Source: CAD feature listing. Evaluate the final solid. Frame: model axes, mm. A direction names the side the tool comes from. Round coordinates to 2 decimals unless told otherwise and drop trailing zeros. Order: outer loops, then holes, each group sorted by start corner. A loop starts at its lowest first (then second) coordinate and runs counter-clockwise, first axis right, second up. Notation, with made-up numbers: M 88,22.25 L 93,22.25 A7 cw 93,32.25 Z; hole C 25,62.5 d1. An arc over 180 degrees is marked long. Answer as CSV lines item,"result". Start each with the question number.
Item 1: Set-up query: faces 4 (the face through (-30, 17.25, -30)), 5 (the face through (22.03, 68.58, 14.04)), 6 (the face through (-16.856, 53.615, 8.767)). Return all of +Z, -Z, +X, -X, +Y, -Y with unobstructed straight access to the full face (end or side cutting, diameter ignored); none if empty.
Item 2: First-contact query: P1, Ø12, axis at x = 35.5, z = 49, coming from the -Y side; P2, Ø4, axis at y = 88.5, z = 22, coming from the -X side; P3, Ø5, axis at x = -16.5, z = 49, coming from the +Y side; P4, Ø3, axis at x = -8.5, y = 46, coming from the +Z side. Flat tips, straight axial feed; report the tip coordinate or a pass-through.
Item 3: Pull-direction query (X, two-part tool) for faces 1 (the face through (8, 128.25, 23)), 2 (the face through (7.1, 119.7, 22.4)), 3 (the face through (35.694, 36.026, -4.686)); classes: +X half, -X half, draft (parallel to the pull), parting line (faces both ways), or undercut.
Item 4: Line query: line 1 (Z direction, x = 0, y = 124) (3 decimals); line 2 (X direction, y = 50, z = 0). Output: solid intervals per line, ascending. Write a range as [from, to].
Item 5: Section query A-A on y = 45. Return the cut outline in (x, z).
from build123d import *

# Parameters (mm, degrees)
F2_R    = 3
F3_R    = 3
F4_SIZE = 1
F5_SIZE = 0.5


with BuildPart() as f1:
    # F0 (on Right) → F1 (revolve)
    with BuildSketch(Plane.YZ):
        Polygon((0, 70), (0, 19), (105.75, 19), (110.25, 23.5), (128.25, 23.5), (128.25, 26.125), (112.25, 26.125), (109.8, 28.575), (73.7, 28.575), (71.25, 26.125), (66.25, 26.125), (52.25, 36), (17.25, 36), (17.25, 70), align=None)
    revolve(axis=Axis((0, 37.063913, 0), (0, 1, 0)))

    # F2
    f2_edges = [f1.edges().sort_by_distance(p)[0] for p in [
        (0, 17.25, -36),
        (0, 66.25, -26.125),
        (0, 71.25, -26.125),
        (0, 112.25, -26.125),
    ]]
    fillet(f2_edges, radius=F2_R)

    # F3
    f3_edges = [f1.edges().sort_by_distance(p)[0] for p in [
        (0, 110.25, -23.5),
    ]]
    fillet(f3_edges, radius=F3_R)

    # F4
    f4_edges = [f1.edges().sort_by_distance(p)[0] for p in [
        (0, 17.25, -70),
    ]]
    chamfer(f4_edges, length=F4_SIZE)

    # F5
    f5_edges = [f1.edges().sort_by_distance(p)[0] for p in [
        (0, 128.25, -26.125),
        (0, 128.25, -23.5),
    ]]
    chamfer(f5_edges, length=F5_SIZE)


solid = f1.part
Results:
1,face 4,"+Y"
1,face 5,"none"
1,face 6,"+Y, -Y"
2,P1,"y = 0"
2,P2,"x = -20.41"
2,P3,"y = 17.25"
2,P4,"z = 35.31"
3,face 1,"draft"
3,face 2,"undercut"
3,face 3,"parting line"
4,line 1,"[-26.125, -23.5], [23.5, 26.125]"
4,line 2,"[-36, -19], [19, 36]"
5,outline,"C 0,0 d72; hole C 0,0 d38"
